```python
from build123d import *

# Parameters (mm, degrees)
SKETCH_2_W             = 60
SKETCH_2_H             = 22
SM_BASE_FLANGE_1_DEPTH = 3
SKETCH_7_W             = 20
SKETCH_7_H             = 2
CUT_EXTRUDE_1_DEPTH    = 30
SKETCH_8_R             = 1.65
CUT_EXTRUDE_2_DEPTH    = 10


# Sheet-metal steps are written as plain solids
with BuildPart() as part:
    # Sketch 2 → 基体-法兰1 (new body)
    with BuildSketch(Plane.XY):
        with Locations((30, 11)):
            Rectangle(SKETCH_2_W, SKETCH_2_H)
    extrude(amount=-SM_BASE_FLANGE_1_DEPTH)

    # 草图7 → 切除-拉伸1 (cut)
    with BuildSketch(Plane.XY):
        with Locations((30, 16)):
            Rectangle(SKETCH_7_W, SKETCH_7_H)
    extrude(amount=-CUT_EXTRUDE_1_DEPTH, mode=Mode.SUBTRACT)

    # 草图8 → 切除-拉伸2 (cut)
    with BuildSketch(Plane.XY):
        with Locations((10, 10)):
            Circle(SKETCH_8_R)
        with Locations((50, 10)):
            Circle(SKETCH_8_R)
    extrude(amount=-CUT_EXTRUDE_2_DEPTH, mode=Mode.SUBTRACT)


solid = part.part
```
Build history of the part. All positions in model axes, mm. A direction names the side the tool comes from. Round coordinates to 2 decimals unless told otherwise and drop trailing zeros. Write each loop counter-clockwise with the first axis right and the second up, starting at its lowest first coordinate (ties: lowest second). Pieces come first, ordered by that corner, then holes. Notation, with made-up numbers: (46.25, -15.5) -> (84.25, -15.5) arc R23 ccw to (84.25, 13.5) -> close; hole circle Ø1 at (35, -25.5). An arc over 180 degrees is marked (long way). Put each result on its own line as item: value.
Item 1: Slice it at D-D, the plane x = 37. Give the cut face in (y, z).
Here are the results:
outline: (0, -3) -> (15, -3) -> (15, 0) -> (0, 0) -> close; (17, -3) -> (22, -3) -> (22, 0) -> (17, 0) -> close
Item 2: Slice it at A-A, the plane x = 50. Give the cut face in (y, z).
Here are the results:
outline: (0, -3) -> (8.35, -3) -> (8.35, 0) -> (0, 0) -> close; (11.65, -3) -> (22, -3) -> (22, 0) -> (11.65, 0) -> close
Item 3: Slice it at B-B, the plane y = 10. Give the cut face in (x, z).
Here are the results:
outline: (0, -3) -> (8.35, -3) -> (8.35, 0) -> (0, 0) -> close; (11.65, -3) -> (48.35, -3) -> (48.35, 0) -> (11.65, 0) -> close; (51.65, -3) -> (60, -3) -> (60, 0) -> (51.65, 0) -> close
Item 4: Tool access for faces 4 (the face through (30, 11, -3)), 5 (the face through (30, 15, -1)): list every direction of +Z, -Z, +X, -X, +Y, -Y with a clear straight run to the whole face (end or side of a thin tool).
Here are the results:
face 4: -Z, +X, -X, +Y, -Y
face 5: +Z, -Z
Item 5: Two-plate mould, pull along Y, no slides. Class faces 1 (the face through (48.69, 9, -1.48)), 2 (the face through (30, 22, -1)), 3 (the face through (60, 11, -1)): pulls with the +Y half, pulls with the -Y half, needs draft (parallel to the pull), parting line crosses it, or undercut.
Here are the results:
face 1: undercut
face 2: pulls with the +Y half
face 3: needs draft
Item 6: Slice it at C-C, the plane z = -0.6. Give the cut face in (x, y).
Here are the results:
outline: (0, 0) -> (60, 0) -> (60, 22) -> (0, 22) -> close; hole circle Ø3.3 at (10, 10); hole (20, 15) -> (40, 15) -> (40, 17) -> (20, 17) -> close; hole circle Ø3.3 at (50, 10)
Item 7: Wall check: probe 1 along Y at (x, z) = (36, -2.9); probe 2 along Y at (x, z) = (10, -1.6); probe 3 along X at (y, z) = (8.5, -0.75). Give the ranges that are in metal, low to high. Write a range as from..to.
Here are the results:
probe 1: y = 0..15, 17..22
probe 2: y = 0..8.35, 11.65..22
probe 3: x = 0..9.31, 10.69..49.31, 50.69..60
